Here's how the part is built. I have some questions about the finished solid (model axes, mm). A direction names the side the tool comes from. Round coordinates to 2 decimals unless told otherwise and drop trailing zeros. Loops run counter-clockwise (first coordinate to the right, second up) from the corner with the lowest first, then second, coordinate; pieces in that order, holes last. Notation, with made-up numbers: M 52.5,71 L 83.5,71 A31 ccw 83.5,100 Z; hole C 3.25,45 d10. An arc over 180 degrees is marked long. Answer as a JSON object with one key per item and string values.
from build123d import *

# Parameters (mm, degrees)
SKETCH1_R           = 9.25
BOSS_EXTRUDE1_DEPTH = 58
SKETCH2_R           = 2.5
BOSS_EXTRUDE2_DEPTH = 1


with BuildPart() as part:
    # Sketch1 → Boss-Extrude1 (new body)
    with BuildSketch(Plane(origin=(0, 0, 0), x_dir=(0, 0, -1), z_dir=(1, 0, 0))):
        with Locations(Location((0, 0, 0), (0, 0, 180))):
            Circle(SKETCH1_R)
    extrude(amount=BOSS_EXTRUDE1_DEPTH)

    # Sketch2 → Boss-Extrude2 (add)
    with BuildSketch(Plane.ZY):
        with Locations(Location((0, 4, 0), (0, 0, 180))):
            Circle(SKETCH2_R)
        with Locations(Location((0, -4, 0), (0, 0, 180))):
            Circle(SKETCH2_R)
    extrude(amount=BOSS_EXTRUDE2_DEPTH)


solid = part.part
Item 1: If I drill on L1, parallel to X at y = -6.5, z = -3.25; L2, parallel to Y at x = 43, z = -2.5; L3, parallel to Z at x = 53.5, y = 4.5, over which ranges is the centre line in solid material (lowest first)? Write a range as from..to.
Solution:
{"L1": "x = 0..58", "L2": "y = -8.91..8.91", "L3": "z = -8.08..8.08"}
Item 2: I want a section at A-A on y = 4. List the corners of the cut face in (x, z) for me, plus the area to 3 significant figures.
Solution:
{"outline": "M -1,-2.5 L 0,-2.5 L 0,-8.34 L 58,-8.34 L 58,8.34 L 0,8.34 L 0,2.5 L -1,2.5 Z", "area": "972 mm2"}
Item 3: For P1, Ø1, axis at y = -5.5, z = 4.5, coming from the -X side; P2, Ø1.5, axis at x = 28, z = 5, coming from the -Y side; P3, Ø1, axis at x = 5.5, z = -6.5, coming from the -Y side, each with a flat end and sliding along its axis, tell me the tip position at first contact or that it passes through.
Solution:
{"P1": "stops at x = 0", "P2": "stops at y = -8.22", "P3": "stops at y = -7.04"}
Item 4: I want a section at C-C on x = 44. List the corners of the cut face in (y, z) for me.
Solution:
{"outline": "C 0,0 d18.5"}
Item 5: We'd pull the mould along Y, two halves only. Please class faces 3 (the face through (-0.49, 1.52, 0.33)), 4 (the face through (58, 0, 0)), 5 (the face through (28.594, 8.206, 4.268)): +Y half, -Y half, draft (parallel to the pull), parting line (faces both ways), or undercut.
Solution:
{"face 3": "undercut", "face 4": "draft", "face 5": "parting line"}
Item 6: For faces 1 (the face through (0, 0, 0)), 2 (the face through (-1, 4, 0)), which set-ups out of +Z, -Z, +X, -X, +Y, -Y let a thin tool reach every point of the face, with its end or its side?
Solution:
{"face 1": "-X", "face 2": "+Z, -Z, -X, +Y, -Y"}
Item 7: I want a section at D-D on y = 0. List the corners of the cut face in (x, z) for me.
Solution:
{"outline": "M 0,-9.25 L 58,-9.25 L 58,9.25 L 0,9.25 Z"}
Item 8: I want a section at B-B on z = -1.75. List the corners of the cut face in (x, y) for me, plus the area to 3 significant figures.
Solution:
{"outline": "M -1,-5.79 L 0,-5.79 L 0,-9.08 L 58,-9.08 L 58,9.08 L 0,9.08 L 0,5.79 L -1,5.79 L -1,2.21 L 0,2.21 L 0,-2.21 L -1,-2.21 Z", "area": "1,060 mm2"}
